Autodesk Inventor part; units mm, degrees
ref_plane "YZ Plane" through (0, 0, 0) normal (1, 0, 0) x (0, 1, 0)
ref_plane "XZ Plane" through (0, 0, 0) normal (0, 1, 0) x (-1, 0, 0)
ref_plane "XY Plane" through (0, 0, 0) normal (0, 0, 1) x (1, 0, 0)
sketch "Skizze1" plane through (0, 0, 0) normal (0, 0, 1) x (1, 0, 0)
  circle A0 centre (0, 0) radius 5
  dimension "d0" = 10
extrude "Extrusion1" add sketch "Skizze1" along normal blind 195
sketch "Skizze2" plane through (0, 0, 195) normal (0, 0, 1) x (1, 0, 0)
  circle A0 centre (0, 0) radius 5
  circle A1 centre (0, 0) radius 7.5
  circle A2 centre (0, 0) radius 5
  line L0 (0, -5) -> (-1.3746, -7.373)
  line L1 (-1.3746, -7.373) -> (-1.8625, -4.6402)
  arc A3 (-1.8625, -4.6402) -> (0, -5) centre (0, 0) ccw
  line L2 (2.1694, -4.5048) -> (1.9606, -7.2392)
  line L3 (1.9606, -7.2392) -> (0.3352, -4.9888)
  arc A4 (0.3352, -4.9888) -> (2.1694, -4.5048) centre (0, 0) ccw
  line L4 (3.9092, -3.1174) -> (4.9074, -5.6716)
  line L5 (4.9074, -5.6716) -> (2.4666, -4.3493)
  arc A5 (2.4666, -4.3493) -> (3.9092, -3.1174) centre (0, 0) ccw
  line L6 (4.8746, -1.1126) -> (6.8822, -2.9807)
  line L7 (6.8822, -2.9807) -> (4.1094, -2.8484)
  arc A6 (4.1094, -2.8484) -> (4.8746, -1.1126) centre (0, 0) ccw
  line L8 (4.8746, 1.1126) -> (7.494, 0.3005)
  line L9 (7.494, 0.3005) -> (4.9383, -0.7833)
  arc A7 (4.9383, -0.7833) -> (4.8746, 1.1126) centre (0, 0) ccw
  line L10 (3.9092, 3.1174) -> (6.6214, 3.5223)
  line L11 (6.6214, 3.5223) -> (4.7891, 1.4369)
  arc A8 (4.7891, 1.4369) -> (3.9092, 3.1174) centre (0, 0) ccw
  line L12 (2.1694, 4.5048) -> (4.4375, 6.0464)
  line L13 (4.4375, 6.0464) -> (3.6914, 3.3725)
  arc A9 (3.6914, 3.3725) -> (2.1694, 4.5048) centre (0, 0) ccw
  line L14 (0, 5) -> (1.3746, 7.373)
  line L15 (1.3746, 7.373) -> (1.8625, 4.6402)
  arc A10 (1.8625, 4.6402) -> (0, 5) centre (0, 0) ccw
  line L16 (-2.1694, 4.5048) -> (-1.9606, 7.2392)
  line L17 (-1.9606, 7.2392) -> (-0.3352, 4.9888)
  arc A11 (-0.3352, 4.9888) -> (-2.1694, 4.5048) centre (0, 0) ccw
  line L18 (-3.9092, 3.1174) -> (-4.9074, 5.6716)
  line L19 (-4.9074, 5.6716) -> (-2.4666, 4.3493)
  arc A12 (-2.4666, 4.3493) -> (-3.9092, 3.1174) centre (0, 0) ccw
  line L20 (-4.8746, 1.1126) -> (-6.8822, 2.9807)
  line L21 (-6.8822, 2.9807) -> (-4.1094, 2.8484)
  arc A13 (-4.1094, 2.8484) -> (-4.8746, 1.1126) centre (0, 0) ccw
  line L22 (-4.8746, -1.1126) -> (-7.494, -0.3005)
  line L23 (-7.494, -0.3005) -> (-4.9383, 0.7833)
  arc A14 (-4.9383, 0.7833) -> (-4.8746, -1.1126) centre (0, 0) ccw
  line L24 (-3.9092, -3.1174) -> (-6.6214, -3.5223)
  line L25 (-6.6214, -3.5223) -> (-4.7891, -1.4369)
  arc A15 (-4.7891, -1.4369) -> (-3.9092, -3.1174) centre (0, 0) ccw
  line L26 (-2.1694, -4.5048) -> (-4.4375, -6.0464)
  line L27 (-4.4375, -6.0464) -> (-3.6914, -3.3725)
  arc A16 (-3.6914, -3.3725) -> (-2.1694, -4.5048) centre (0, 0) ccw
  dimension "d3" = 15
  dimension "d6" = 360
extrude "Extrusion2" add sketch "Skizze2" along normal blind 7 contours A0 | A0 L8 L9 | A0 L10 L11 | L6 L7 A0 | A0 L12 L13 | L4 L5 A0 | L15 A0 L14 | L3 A0 L2 | L17 A0 L16 | L1 A0 L0 | L19 A0 L18 | L27 A0 L26 | L21 A0 L20 | L25 A0 L24 | L23 A0 L22
ref_plane "Arbeitsebene1" through (0, 0, 97.5) normal (0, 0, -1) x (-1, 0, 0)
mirror "Spiegeln2" about plane through (0, 0, 97.5) normal (0, 0, -1) of "Extrusion2"
equation "\"d0\" = Durchmesser3"
equation "\"d3\" = Durchmesser1"
equation "\"Durchmesser1\" = 15"
equation "\"Größe1\" = 7"
equation "\"Durchmesser2\" = 3"
equation "\"Durchmesser3\" = 10"
equation "\"Größe3\" = 3"
equation "\"Größe4\" = 15"
properties part number "WelleRuder2"
Can you work these out from the model? Positions are in its coordinate system, mm. Give positions to 0.01 mm unless a question says otherwise; leave off trailing zeros. Order: outer loops, then holes, each group sorted by start corner. A loop starts at its lowest first (then second) coordinate and runs counter-clockwise, first axis right, second up. Notation, with made-up numbers: M 14,66 L 69,66 A9 ccw 69,82 Z; hole C 12.25,21.25 d8. An arc over 180 degrees is marked long. Write item = value, one per line. Start each with the question number.
Q1. I need wall thicknesses on probe 1 along Z at (x, y) = (-1.25, 6); probe 2 along Y at (x, z) = (4, 51.5); probe 3 along X at (y, z) = (0.25, 106). Which ranges of each line are inside material? Lowest first, please. Write a range as [from, to].
Q2. We'd pull the mould along Z, two halves only. Please class faces 1 (the cylindrical face through (-1.08, 4.88, 96.04)), 2 (the flat face through (0, 0, 202)), 3 (the flat face through (0, 0, -7)): pulls with the +Z half, pulls with the -Z half, needs draft (parallel to the pull), parting line crosses it, or undercut.
Q3. Suppose I cut it at A-A (z = 129). Write out the boundary of the cut face in (x, y), plus the area to 3 significant figures.
Q4. Will these pins go through, and if not, where does the flat tip stop? pin 1 Ø2 at (y, z) = (-3, 23) entering from -X; pin 2 Ø3 at (y, z) = (-6, 61) entering from -X; pin 3 Ø2 at (y, z) = (4, 25) entering from +X.
Check result:
q1.probe_1 = [-7, 0], [195, 202]
q1.probe_2 = [-3, 3]
q1.probe_3 = [-4.99, 4.99]
q2.face_1 = undercut
q2.face_2 = pulls with the +Z half
q2.face_3 = pulls with the -Z half
q3.outline = C 0,0 d10
q3.area = 78.5 mm2
q4.pin_1 = -4.58
q4.pin_2 = -2.18
q4.pin_3 = 4
